Geometry check sheet. Reference: the model listing, model coordinates, mm. Round coordinates to 2 decimals unless told otherwise and drop trailing zeros. Write each loop counter-clockwise with the first axis right and the second up, starting at its lowest first coordinate (ties: lowest second). Pieces come first, ordered by that corner, then holes.
Item 1: Scan lines: probe 1 along Y at (x, z) = (0, -83.25); probe 2 along X at (y, z) = (-1.25, -6.5); probe 3 along Z at (x, y) = (1.75, 1). Record each from-to range of solid material in increasing order.
Item 2: Depth check by flat-ended pin: P1, Ø2, axis at y = -1.5, z = -30, coming from the +X side; P2, Ø2, axis at x = 2, z = -27.5, coming from the -Y side. Enter the tip coordinate at first touch or a pass-through.
Item 3: Cross-section at A-A (z = -29). Enter the section's corners in (x, y).
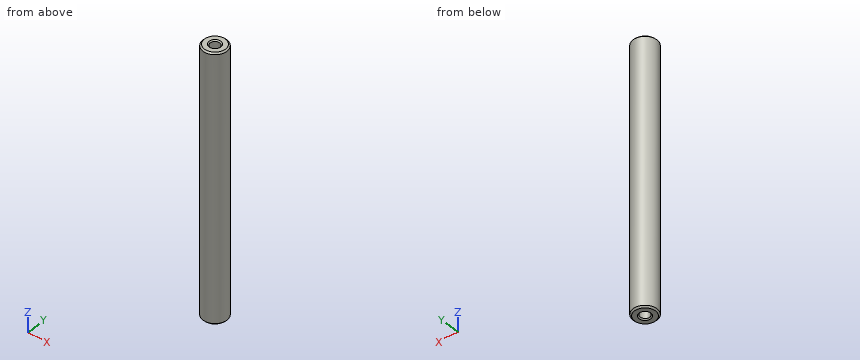
from build123d import *

# Parameters (mm, degrees)
SKETCH1_R                  = 4.1
BLANK_DEPTH                = 91
FURO_1_M4X11_5_D           = 3.3
FURO_1_M4X11_5_DEPTH       = 10.508579979
FURO_1_M4X11_5_CSINK_D     = 4.05
FURO_1_M4X11_5_CSINK_ANGLE = 90
FURO_1_M4X11_5_TIP         = 0.991420021
FURO_2_M4X11_5_D           = 3.3
FURO_2_M4X11_5_DEPTH       = 10.508579979
FURO_2_M4X11_5_CSINK_D     = 4.05
FURO_2_M4X11_5_CSINK_ANGLE = 90
FURO_2_M4X11_5_TIP         = 0.991420021
CHANFROS_SIZE              = 0.5


with BuildPart() as part:
    # Sketch1 → Blank (new body)
    with BuildSketch(Plane.XY):
        Circle(SKETCH1_R)
    extrude(amount=-BLANK_DEPTH)

    # Furo 1 -  M4x11.5
    with Locations(Plane.XY):
        with Locations((0, 0)):
            CounterSinkHole(FURO_1_M4X11_5_D / 2, FURO_1_M4X11_5_CSINK_D / 2, depth=FURO_1_M4X11_5_DEPTH, counter_sink_angle=FURO_1_M4X11_5_CSINK_ANGLE)
            with Locations((0, 0, -(FURO_1_M4X11_5_DEPTH + FURO_1_M4X11_5_TIP / 2))):  # 118° drill point
                Cone(0, FURO_1_M4X11_5_D / 2, FURO_1_M4X11_5_TIP, mode=Mode.SUBTRACT)

    # Furo 2 -  M4x11.5
    with Locations(Plane(origin=(0, 0, -91), x_dir=(-1, 0, 0), z_dir=(0, 0, -1))):
        with Locations((0, 0)):
            CounterSinkHole(FURO_2_M4X11_5_D / 2, FURO_2_M4X11_5_CSINK_D / 2, depth=FURO_2_M4X11_5_DEPTH, counter_sink_angle=FURO_2_M4X11_5_CSINK_ANGLE)
            with Locations((0, 0, -(FURO_2_M4X11_5_DEPTH + FURO_2_M4X11_5_TIP / 2))):  # 118° drill point
                Cone(0, FURO_2_M4X11_5_D / 2, FURO_2_M4X11_5_TIP, mode=Mode.SUBTRACT)

    # Chanfros
    chanfros_edges = [part.edges().sort_by_distance(p)[0] for p in [
        (-4.1, 0, 0),
        (-4.1, 0, -91),
    ]]
    chamfer(chanfros_edges, length=CHANFROS_SIZE)


solid = part.part
Resolved:
1. probe 1: y = -4.1 to -1.65, 1.65 to 4.1
1. probe 2: x = -3.9 to -1.08, 1.08 to 3.9
1. probe 3: z = -90.99 to -0.01
2. P1: stops at x = 4.07
2. P2: stops at y = -3.98
3. outline: circle Ø8.2 at (0, 0)
